Model file for the job. Use its own axes, mm. A direction names the side the tool comes from. Coordinates: 2 decimals unless noted, no trailing zeros. Write each loop counter-clockwise with the first axis right and the second up, starting at its lowest first coordinate (ties: lowest second). Pieces come first, ordered by that corner, then holes. Notation, with made-up numbers: M -14.5,-30.5 L 3.5,-30.5 A26 cw 3.5,-5.5 Z; hole C 10.25,46 d1. An arc over 180 degrees is marked long. One line per question, with ' | ' between items. Start each with the question number.
(1) Cut at B-B (x = 0). Write the cut outline in (y, z).
(2) Two-plate mould, pull along X, no slides. Class faces 1 (the face through (-14.78, -15.73, 22.23)), 2 (the face through (0, 0, 30)), 3 (the face through (15.795, 0.266, 15.21)): +X half, -X half, draft (parallel to the pull), parting line (faces both ways), or undercut.
(3) Tool access for faces 4 (the face through (2.4, 15.7, 16.8)), 5 (the face through (14.76, 16.16, 22.23)): list every direction of +Z, -Z, +X, -X, +Y, -Y with a clear straight run to the whole face (end or side of a thin tool).
(4) Flat gauge pins, fed straight in: pin 1 Ø6 at (y, z) = (-10, 13) entering from +X; pin 2 Ø2 at (x, y) = (-16, 16) entering from +Z; pin 3 Ø8 at (y, z) = (-1.5, 13) entering from +X; pin 4 Ø3 at (y, z) = (12, 24.5) entering from -X. Where does each tip first touch, or does it go through?
(5) Cut at A-A (y = -12.5). Write the cut outline in (x, z), plus the area to 3 significant figures.
(6) Cut at C-C (z = 13). Write the cut outline in (x, y).
(7) Cut at D-D (z = 26). Write the cut outline in (x, y), plus the area to 3 significant figures.
(8) Wall check: probe 1 along Y at (x, z) = (-16, 23.5); probe 2 along Y at (x, z) = (0, 0.85); probe 3 along X at (y, z) = (-16, 23.75). Give the ranges that are in metal, low to high.
Autodesk Inventor part; units mm, degrees
ref_plane "YZ Plane" through (0, 0, 0) normal (1, 0, 0) x (0, 1, 0)
ref_plane "XZ Plane" through (0, 0, 0) normal (0, 1, 0) x (-1, 0, 0)
ref_plane "XY Plane" through (0, 0, 0) normal (0, 0, 1) x (1, 0, 0)
sketch "Sketch1" plane through (0, 0, 0) normal (0, 0, 1) x (1, 0, 0)
  line L0 (12.5, -19) -> (-12.5, -19)
  line L1 (-12.5, -19) -> (-12.5, 19)
  line L2 (-12.5, 19) -> (12.5, 19)
  line L3 (12.5, 19) -> (12.5, -19)
  line L4 (12.5, -19) -> (-12.5, 19) construction
  line L5 (-12.5, -19) -> (12.5, 19) construction
  circle A0 centre (0, 12.5) radius 2.1
  circle A1 centre (0, -12.5) radius 2.1
  point P0 (0, 0)
  dimension "d0" = 25
  dimension "d1" = 38
  dimension "d2" = 4.2
  dimension "d3" = 4.2
  dimension "d4" = 12.5
  dimension "d5" = 12.5
extrude "Extrusion1" add sketch "Sketch1" along normal blind 30
sketch "Sketch2" plane through (-12.5, 19, 0) normal (0, 1, 0) x (1, 0, 0)
  line L0 (0, 0) -> (0, -30)
  line L1 (0, -30) -> (-6.5, -30)
  line L2 (-6.5, -30) -> (0, 0)
  line L3 (0, -30) -> (25, -30)
  line L4 (0, 0) -> (0, -30)
  line L5 (25, -30) -> (31.5, -30)
  line L6 (25, 0) -> (25, -30)
  line L7 (31.5, -30) -> (25, 0)
  line L8 (25, 0) -> (25, -30)
  point P0 (12.5, 0)
  dimension "d8" = 6.5
  dimension "d9" = 6.5
extrude "Extrusion2" add sketch "Sketch2" against normal up to surface (38 mm away)
sketch "Sketch3" plane through (0, 0, 30) normal (0, 0, 1) x (1, 0, 0)
  line L0 (-5.4088, 0) -> (7.7062, 0)
  line L1 (0, 5.8117) -> (0, -6.6687)
  point P0 (0, 0)
  point P1 (-16, 16)
  point P2 (16, 16)
  point P3 (-16, -16)
  point P4 (16, -16)
  dimension "d12" = 16
  dimension "d13" = 16
  dimension "d16" = 32
  dimension "d19" = 32
hole "Hole1" at (-16, 16, 30) at (16, 16, 30) at (-16, -16, 30) at (16, -16, 30) direction (0, 0, -1) diameter 2.5 depth 20 tip angle 118
hole "Hole2" at (0, -12.5, 30) direction (0, 0, -1) diameter 8 depth 26 tip angle 118
hole "Hole3" at (0, 12.5, 30) direction (0, 0, -1) diameter 8 depth 26 tip angle 118
properties part number "RDtoRC2-height30mm"
Filled in:
1) outline: M -19,0 L -14.6,0 L -14.6,2.86 L -16.5,4 L -16.5,30 L -19,30 Z; M -10.4,0 L 10.4,0 L 10.4,2.86 L 8.5,4 L 8.5,30 L -8.5,30 L -8.5,4 L -10.4,2.86 Z; M 14.6,0 L 19,0 L 19,30 L 16.5,30 L 16.5,4 L 14.6,2.86 Z
2) face 1: undercut | face 2: draft | face 3: +X half
3) face 4: +Z | face 5: +Z, -Z
4) pin 1: x = 15.97 | pin 2: through | pin 3: x = 16.18 | pin 4: x = -18.13
5) outline: M -19,30 L -12.5,0 L -2.1,0 L -2.1,2.86 L -4,4 L -4,30 Z; M 2.1,0 L 12.5,0 L 19,30 L 4,30 L 4,4 L 2.1,2.86 Z | area: 718 mm²
6) outline: M -15.32,-19 L 15.32,-19 L 15.32,-17.05 A1.25 cw 15.32,-14.95 L 15.32,14.95 A1.25 cw 15.32,17.05 L 15.32,19 L -15.32,19 L -15.32,17.05 A1.25 cw -15.32,14.95 L -15.32,-14.95 A1.25 cw -15.32,-17.05 Z; hole C 0,-12.5 d8; hole C 0,12.5 d8
7) outline: M -18.13,-19 L 18.13,-19 L 18.13,19 L -18.13,19 Z; hole C -16,-16 d2.5; hole C -16,16 d2.5; hole C 0,-12.5 d8; hole C 0,12.5 d8; hole C 16,-16 d2.5; hole C 16,16 d2.5 | area: 1,260 mm²
8) probe 1: -19 to -17.25, -14.75 to 14.75, 17.25 to 19 | probe 2: -19 to -14.6, -10.4 to 10.4, 14.6 to 19 | probe 3: -17.65 to -17.25, -14.75 to -1.94, 1.94 to 14.75, 17.25 to 17.65
